The model under review builds one solid part; all positions refer to its coordinate system, in mm. Face numbers are marked on the shaded views. A direction names the side the tool comes from. Coordinates: 2 decimals unless noted, no trailing zeros. Write each loop counter-clockwise with the first axis right and the second up, starting at its lowest first coordinate (ties: lowest second). Pieces come first, ordered by that corner, then holes. Notation, with made-up numbers: (-38, 2) - (16, 2) arc R9 cw to (16, 6) - close; hole circle Ø3 at (71.25, -9). An arc over 180 degrees is marked (long way). Return JSON: item names as keys, results as strings. Group by question number.
(1) We need section C-C on x = 1.75. State the section outline as (y, z) points, then the cut area to 3 significant figures.
(2) Tool access review of the marked faces 4, 5, 6, 7 and 8: name each direction out of +Z, -Z, +X, -X, +Y, -Y from which nothing blocks a thin tool from reaching the whole face with its end or side.
(3) We need section A-A on y = -28.95. State the section outline as (x, z) points.
(4) For pin 1 Ø1 at (x, y) = (-14.5, -18) entering from +Z; pin 2 Ø10 at (y, z) = (-23, 14) entering from +X; pin 3 Ø8 at (x, z) = (-10.5, 7) entering from -Y, all flat-tipped, find the tip position at first contact; note any pin that passes through.
(5) We need section D-D on y = -24.25. State the section outline as (x, z) points.
(6) To check wall thickness, follow L1, parallel to Y at x = -0.75, z = 27; L2, parallel to Y at x = -11.5, z = 16.5; L3, parallel to X at y = -11, z = 7.5. State the ranges of each line that lie inside material, in increasing order. Write a range as from..to.
(7) We need section B-B on x = -13.5. State the section outline as (y, z) points, then the cut area to 4 significant figures.
(8) Draft analysis for pull direction Z (two halves, no side actions). For the marked faces 1, 2 and 3, state which applies: released by +Z, released by -Z, zero draft, split by the parting line, or undercut.
```python
from build123d import *

# Parameters (mm, degrees)
SKETCH1_W                      = 27
SKETCH1_H                      = 29
BOSS_EXTRUDE1_DEPTH            = 2
SKETCH4_W                      = 10
SKETCH4_H                      = 29
BOSS_EXTRUDE3_DEPTH            = 2
BOSS_EXTRUDE4_DEPTH            = 29
SKETCH6_R                      = 1.65
CUT_EXTRUDE1_DEPTH             = 2
CHAMFER1_SIZE                  = 1
SKETCH7_W                      = 23
SKETCH7_H                      = 7
CUT_EXTRUDE3_DEPTH             = 2
CUT_EXTRUDE3_DIRECTION_2_REACH = 48.872
BOSS_EXTRUDE6_REACH            = 49.938
SKETCH9_W                      = 28
SKETCH9_H                      = 9
SKETCH9_W_2                    = 23
SKETCH9_H_2                    = 7
CHAMFER3_SIZE                  = 2
SKETCH10_R                     = 1.65
CUT_EXTRUDE4_DEPTH             = 10
SKETCH11_W                     = 2.8
SKETCH11_H                     = 2.9
BOSS_EXTRUDE7_DEPTH            = 3


with BuildPart() as part:
    # Sketch1 → Boss-Extrude1 (new body)
    with BuildSketch(Plane.XY):
        with Locations((-3.250075758, -20.95)):
            Rectangle(SKETCH1_W, SKETCH1_H)
    extrude(amount=BOSS_EXTRUDE1_DEPTH)

    # Sketch4 → Boss-Extrude3 (add)
    with BuildSketch(Plane.ZY.offset(16.750075758)):
        with Locations((5, -20.95)):
            Rectangle(SKETCH4_W, SKETCH4_H)
    extrude(amount=BOSS_EXTRUDE3_DEPTH)

    # Sketch5 → Boss-Extrude4 (add)
    with BuildSketch(Plane.XZ.offset(35.45)):
        Polygon((-18.750075758, 10), (-2.48661979, 26.263455967), (-1.48661979, 25.263455967), (-16.750075758, 10), align=None)
    extrude(amount=-BOSS_EXTRUDE4_DEPTH)

    # Sketch6 → Cut-Extrude1 (cut)
    with BuildSketch(Plane(origin=(-13.375037879, 0, 13.375037879), x_dir=(-0.7071067811865435, 0, -0.7071067811865517), z_dir=(0.7071067811865517, 0, -0.7071067811865435))):
        with Locations((-11.812762096, -32.45)):
            Circle(SKETCH6_R)
        with Locations((-11.812762096, -18.45)):
            Circle(SKETCH6_R)
    extrude(amount=-CUT_EXTRUDE1_DEPTH, mode=Mode.SUBTRACT)

    # Chamfer1
    chamfer1_edges = [part.edges().sort_by_distance(p)[0] for p in [
        (-16.750075758, -20.95, 2),
    ]]
    chamfer(chamfer1_edges, length=CHAMFER1_SIZE)

    # Sketch7 → Cut-Extrude3 (cut)
    with BuildSketch(Plane.XY.offset(2)):
        with Locations((-3.250075758, -10.95)):
            Rectangle(SKETCH7_W, SKETCH7_H)
    extrude(amount=-CUT_EXTRUDE3_DEPTH, mode=Mode.SUBTRACT)

    # Cut-Extrude3 direction 2: up to this plane
    cut_extrude3_direction_2_end = Plane(origin=(-18.750075758, 17.267649798, 10), z_dir=(-0.7071067811865512, 0, 0.7071067811865439))
    # Sketch7 → Cut-Extrude3 direction 2 (cut, up to the surface)
    with BuildSketch(Plane.XY.offset(2), mode=Mode.PRIVATE) as cut_extrude3_direction_2_sk1:
        with Locations((-3.250075758, -10.95)):
            Rectangle(SKETCH7_W, SKETCH7_H)
    cut_extrude3_direction_2_tool1 = split(extrude(cut_extrude3_direction_2_sk1.sketch, amount=CUT_EXTRUDE3_DIRECTION_2_REACH, mode=Mode.PRIVATE), bisect_by=cut_extrude3_direction_2_end, keep=Keep.BOTH, mode=Mode.PRIVATE)
    add(cut_extrude3_direction_2_tool1.solids().sort_by_distance((-3.250076, -10.95, 2))[0], mode=Mode.SUBTRACT)

    # Boss-Extrude6: up to this plane
    boss_extrude6_end = Plane(origin=(-18.750075758, 17.267649798, 10), z_dir=(-0.7071067811865512, 0, 0.7071067811865439))
    # Sketch9 → Boss-Extrude6 (add, up to the surface)
    with BuildSketch(Plane(origin=(0, 0, 0), x_dir=(-1, 0, 0), z_dir=(0, 0, -1)), mode=Mode.PRIVATE) as boss_extrude6_sk1:
        with Locations((4.750075758, -10.95)):
            Rectangle(SKETCH9_W, SKETCH9_H)
        with Locations((3.250075758, -10.95)):
            Rectangle(SKETCH9_W_2, SKETCH9_H_2, mode=Mode.SUBTRACT)
    boss_extrude6_tool1 = split(extrude(boss_extrude6_sk1.sketch, amount=-BOSS_EXTRUDE6_REACH, mode=Mode.PRIVATE), bisect_by=boss_extrude6_end, keep=Keep.BOTH, mode=Mode.PRIVATE)
    add(boss_extrude6_tool1.solids().sort_by_distance((-4.750076, -15.155891, 0))[0])

    # Chamfer3
    chamfer3_edges = [part.edges().sort_by_distance(p)[0] for p in [
        (-18.750075758, -20.95, 0),
    ]]
    chamfer(chamfer3_edges, length=CHAMFER3_SIZE)

    # Sketch10 → Cut-Extrude4 (cut)
    with BuildSketch(Plane.XY.offset(2)):
        with Locations((1.249924242, -28.95)):
            Circle(SKETCH10_R)
    extrude(amount=-CUT_EXTRUDE4_DEPTH, mode=Mode.SUBTRACT)

    # Sketch11 → Boss-Extrude7 (add)
    with BuildSketch(Plane(origin=(0, 0, 0), x_dir=(-1, 0, 0), z_dir=(0, 0, -1))):
        with Locations((-4.749924242, -15.9)):
            Rectangle(SKETCH11_W, SKETCH11_H)
        with Locations((11.250075758, -15.9)):
            Rectangle(SKETCH11_W, SKETCH11_H)
    extrude(amount=BOSS_EXTRUDE7_DEPTH)


solid = part.part
```
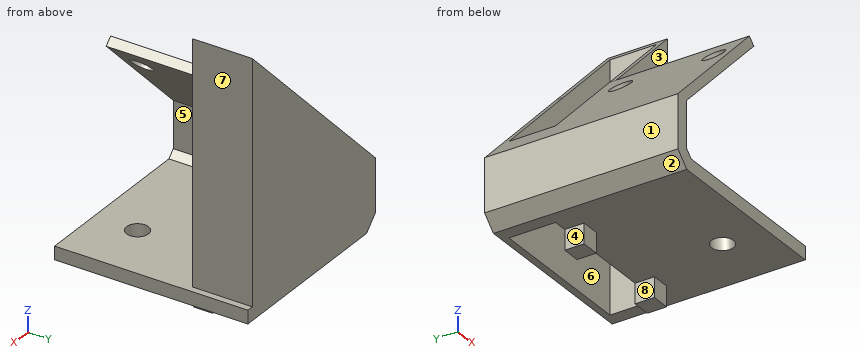
Ans:
{
 "1": {"outline": "(-35.45, 0) - (-30.52, 0) - (-30.52, 2) - (-35.45, 2) - close; (-27.38, 0) - (-14.45, 0) - (-14.45, 30.5) - (-15.45, 30.5) - (-15.45, 2) - (-27.38, 2) - close; (-7.45, 0) - (-6.45, 0) - (-6.45, 30.5) - (-7.45, 30.5) - close", "area": "94.7 mm²"},
 "2": {"face 4": "-Z, -X, +Y, -Y", "face 5": "+X, -Y", "face 6": "+Z, -Z", "face 7": "+Z, +X, +Y, -Y", "face 8": "-Z, +Y, -Y"},
 "3": {"outline": "(-18.75, 2) - (-16.75, 0) - (-0.4, 0) - (-0.4, 2) - (-15.75, 2) - (-16.75, 3) - (-16.75, 10) - (-1.49, 25.26) - (-2.49, 26.26) - (-18.75, 10) - close; (2.9, 0) - (10.25, 0) - (10.25, 2) - (2.9, 2) - close"},
 "4": {"pin 1": "z = 14.75", "pin 2": "x = -7.75", "pin 3": "y = -15.45"},
 "5": {"outline": "(-18.75, 2) - (-16.75, 0) - (10.25, 0) - (10.25, 2) - (-15.75, 2) - (-16.75, 3) - (-16.75, 10) - (-1.49, 25.26) - (-2.49, 26.26) - (-18.75, 10) - close"},
 "6": {"L1": "-15.45..-14.45, -7.45..-6.45", "L2": "-35.45..-14.45, -7.45..-6.45", "L3": "-18.75..-14.75, 8.25..9.25"},
 "7": {"outline": "(-35.45, 0) - (-14.45, 0) - (-14.45, 15.25) - (-35.45, 15.25) - (-35.45, 13.25) - (-15.45, 13.25) - (-15.45, 2) - (-35.45, 2) - close; (-7.45, 0) - (-6.45, 0) - (-6.45, 15.25) - (-7.45, 15.25) - close", "area": "110.5 mm²"},
 "8": {"face 1": "zero draft", "face 2": "released by -Z", "face 3": "undercut"}
}
